from build123d import *
from build123d.topology import SkipClean

# Parameters (mm, degrees)
SKETCH3_W               = 29
SKETCH3_H               = 29
SKETCH3_R               = 1.2
SKETCH3_W_2             = 5
SKETCH3_H_2             = 6
BOSS_EXTRUDE1_DEPTH     = 5
SKETCH4_W               = 29
SKETCH4_H               = 42
SKETCH4_W_2             = 20
SKETCH4_H_2             = 11
BOSS_EXTRUDE2_DEPTH     = 10
BOSS_EXTRUDE3_START     = 3
SKETCH5_W               = 6
SKETCH5_H               = 6
SKETCH5_R               = 1.2
BOSS_EXTRUDE3_DEPTH     = 3
FILLET1_DEPTH           = 22
FILLET1_START           = 19.5
FILLET1_2_DEPTH         = 9.5
FILLET1_3_DEPTH         = 9.5
FILLET1_START_2         = 27
FILLET1_4_DEPTH         = 2
FILLET1_START_3         = 12.5
FILLET1_5_DEPTH         = 4
FILLET1_START_4         = 5
FILLET1_6_OUTLINE_R     = 1.2
FILLET1_6_DEPTH         = 20
CUT_EXTRUDE1_DEPTH      = 47.540305175
CUT_EXTRUDE1_DEPTH_BACK = 2
FILLET2_R               = 1
SKETCH7_R               = 2.05
CUT_EXTRUDE2_DEPTH      = 49.031239886
FILLET3_R               = 2


with BuildPart() as part:
    # Sketch3 → Boss-Extrude1 (new body)
    with BuildSketch(Plane.XY):
        with Locations((14.5, 14.5)):
            Rectangle(SKETCH3_W, SKETCH3_H)
        with Locations((3, 26)):
            Circle(SKETCH3_R, mode=Mode.SUBTRACT)
        with Locations(Location((26, 26, 0), (0, 0, 180))):
            Circle(SKETCH3_R, mode=Mode.SUBTRACT)
        with Locations((26, 3)):
            Circle(SKETCH3_R, mode=Mode.SUBTRACT)
        with Locations(Location((3, 3, 0), (0, 0, 180))):
            Circle(SKETCH3_R, mode=Mode.SUBTRACT)
        with Locations((24.5, 9)):
            Rectangle(SKETCH3_W_2, SKETCH3_H_2, mode=Mode.SUBTRACT)
        with BuildLine():
            Line((16.5, 7), (16.5, 22))
            ThreePointArc((16.5, 22), (18, 23.5), (19.5, 22))
            Line((19.5, 22), (19.5, 7))
            ThreePointArc((19.5, 7), (18, 5.5), (16.5, 7))
        make_face(mode=Mode.SUBTRACT)
        with BuildLine():
            Line((12.5, 7), (12.5, 22))
            ThreePointArc((12.5, 22), (11, 23.5), (9.5, 22))
            Line((9.5, 22), (9.5, 7))
            ThreePointArc((9.5, 7), (11, 5.5), (12.5, 7))
        make_face(mode=Mode.SUBTRACT)
    extrude(amount=BOSS_EXTRUDE1_DEPTH)

    # Sketch4 → Boss-Extrude2 (add)
    with BuildSketch(Plane(origin=(0, 0, 0), x_dir=(1, 0, 0), z_dir=(0, 1, 0))):
        with Locations((14.5, -4)):
            Rectangle(SKETCH4_W, SKETCH4_H)
        with Locations((14.5, 2.5)):
            Rectangle(SKETCH4_W_2, SKETCH4_H_2, mode=Mode.SUBTRACT)
    extrude(amount=-BOSS_EXTRUDE2_DEPTH)

    # Sketch5 → Boss-Extrude3 (add)
    # profile 1 of 4: a face of its own
    with BuildSketch(Plane(origin=(0, 0, 0), x_dir=(-1, 0, 0), z_dir=(0, 0, -1)).offset(BOSS_EXTRUDE3_START)):
        with Locations((-26, 3)):
            Rectangle(SKETCH5_W, SKETCH5_H)
        with Locations((-26, 3)):
            Circle(SKETCH5_R, mode=Mode.SUBTRACT)
    # profile 2 of 4: a face of its own
    with BuildSketch(Plane(origin=(0, 0, 0), x_dir=(-1, 0, 0), z_dir=(0, 0, -1)).offset(BOSS_EXTRUDE3_START)):
        with Locations((-26, 26)):
            Rectangle(SKETCH5_W, SKETCH5_H)
        with Locations((-26, 26)):
            Circle(SKETCH5_R, mode=Mode.SUBTRACT)
    # profile 3 of 4: a face of its own
    with BuildSketch(Plane(origin=(0, 0, 0), x_dir=(-1, 0, 0), z_dir=(0, 0, -1)).offset(BOSS_EXTRUDE3_START)):
        with Locations((-3, 3)):
            Rectangle(SKETCH5_W, SKETCH5_H)
        with Locations((-3, 3)):
            Circle(SKETCH5_R, mode=Mode.SUBTRACT)
    # profile 4 of 4: a face of its own
    with BuildSketch(Plane(origin=(0, 0, 0), x_dir=(-1, 0, 0), z_dir=(0, 0, -1)).offset(BOSS_EXTRUDE3_START)):
        with Locations((-3, 26)):
            Rectangle(SKETCH5_W, SKETCH5_H)
        with Locations((-3, 26)):
            Circle(SKETCH5_R, mode=Mode.SUBTRACT)
    extrude(amount=-BOSS_EXTRUDE3_DEPTH)

    # Fillet1: read off the stored shape, not the designer's step
    # Fillet1 outline → Fillet1 (add)
    with BuildSketch(Plane.YZ):
        with BuildLine():
            Line((12, 5), (12, 6.66969722))
            ThreePointArc((12, 6.66969722), (3.266799469, 14.04554885), (0, 25))
            Line((0, 25), (0, 5))
            Line((0, 5), (12, 5))
        make_face()
    extrude(amount=FILLET1_DEPTH)

    # Fillet1 2 outline → Fillet1 2 (add)
    with SkipClean():  # the faces are left unmerged after this step: merging them gives an invalid solid
        with BuildSketch(Plane.YZ.offset(FILLET1_START)):
            with BuildLine():
                ThreePointArc((20, 5), (15.913807126, 5.421873741), (12, 6.66969722))
                Line((12, 6.66969722), (12, 5))
                Line((12, 5), (20, 5))
            make_face()
            with BuildLine():
                Line((6, 5), (6, 10.717143143))
                ThreePointArc((6, 10.717143143), (1.560911085, 17.254033307), (0, 25))
                Line((0, 25), (0, 5))
                Line((0, 5), (6, 5))
            make_face()
        extrude(amount=FILLET1_2_DEPTH)
    add(part.part.scale(1), mode=Mode.REPLACE)  # the faces are merged on a copy

    # Fillet1 3 outline → Fillet1 3 (add)
    with BuildSketch(Plane.YZ):
        with BuildLine():
            ThreePointArc((20, 5), (15.913807126, 5.421873741), (12, 6.66969722))
            Line((12, 6.66969722), (12, 5))
            Line((12, 5), (20, 5))
        make_face()
    extrude(amount=FILLET1_3_DEPTH)

    # Fillet1 4 outline → Fillet1 4 (add)
    with BuildSketch(Plane.YZ.offset(FILLET1_START_2)):
        with BuildLine():
            Line((12, 5), (12, 6.66969722))
            ThreePointArc((12, 6.66969722), (8.815392066, 8.419754363), (6, 10.717143143))
            Line((6, 10.717143143), (6, 5))
            Line((6, 5), (12, 5))
        make_face()
    extrude(amount=FILLET1_4_DEPTH)

    # Fillet1 5 outline → Fillet1 5 (add)
    with SkipClean():  # the faces are left unmerged after this step: merging them gives an invalid solid
        with BuildSketch(Plane.YZ.offset(FILLET1_START_3)):
            with BuildLine():
                ThreePointArc((20, 5), (15.913807126, 5.421873741), (12, 6.66969722))
                Line((12, 6.66969722), (12, 5))
                Line((12, 5), (20, 5))
            make_face()
        extrude(amount=FILLET1_5_DEPTH)

    # Fillet1 6 outline → Fillet1 6 (cut)
    with BuildSketch(Plane.XY.offset(FILLET1_START_4)):
        with Locations((26, 3)):
            Circle(FILLET1_6_OUTLINE_R)
        with Locations((3, 3)):
            Circle(FILLET1_6_OUTLINE_R)
        with BuildLine():
            ThreePointArc((16.5, 7), (18, 5.5), (19.5, 7))
            Line((19.5, 7), (19.5, 12))
            Line((19.5, 12), (16.5, 12))
            Line((16.5, 12), (16.5, 7))
        make_face()
        with BuildLine():
            ThreePointArc((9.5, 7), (11, 5.5), (12.5, 7))
            Line((12.5, 7), (12.5, 12))
            Line((12.5, 12), (9.5, 12))
            Line((9.5, 12), (9.5, 7))
        make_face()
    extrude(amount=FILLET1_6_DEPTH, mode=Mode.SUBTRACT)

    # Sketch6 → Cut-Extrude1 (cut, two sides: drawn at the far end of the back side and taken through both)
    with BuildSketch(Plane.XY.offset(5).offset(-CUT_EXTRUDE1_DEPTH_BACK)):
        Polygon((4.385640646, 0.6), (5.771281292, 3), (4.385640646, 5.4), (1.614359354, 5.4), (0.228718708, 3), (1.614359354, 0.6), align=None)
        Polygon((24.614359354, 0.6), (27.385640646, 0.6), (28.771281292, 3), (27.385640646, 5.4), (24.614359354, 5.4), (23.228718708, 3), align=None)
        Polygon((4.385640646, 23.6), (5.771281292, 26), (4.385640646, 28.4), (1.614359354, 28.4), (0.228718708, 26), (1.614359354, 23.6), align=None)
        Polygon((27.385640646, 23.6), (28.771281292, 26), (27.385640646, 28.4), (24.614359354, 28.4), (23.228718708, 26), (24.614359354, 23.6), align=None)
    extrude(amount=CUT_EXTRUDE1_DEPTH + CUT_EXTRUDE1_DEPTH_BACK, mode=Mode.SUBTRACT)

    # Fillet2
    fillet2_edges = [part.edges().sort_by_distance(p)[0] for p in [
        (28, 6, 0),
        (26, 23, 0),
        (3, 23, 0),
        (3, 6, 0),
        (6, 3, 0),
        (6, 26, 0),
        (23, 26, 0),
        (23, 3, 0),
    ]]
    fillet(fillet2_edges, radius=FILLET2_R)

    # Sketch7 → Cut-Extrude2 (cut, through all)
    with BuildSketch(Plane.ZY):
        with Locations((-13, -5)):
            Circle(SKETCH7_R)
        with Locations((17, -5)):
            Circle(SKETCH7_R)
    extrude(amount=-CUT_EXTRUDE2_DEPTH, mode=Mode.SUBTRACT)

    # Fillet3
    # the kernel refuses this fillet: 2 mm, written as the material it takes off along each edge
    with BuildSketch(Plane(origin=(-5, -10, -17), x_dir=(0, 0, 1), z_dir=(1, 0, 0)), Plane(origin=(34, -10, 25), x_dir=(0, 0, -1), z_dir=(-1, 0, 0))) as fillet3_piece_1:
        with BuildLine():
            CenterArc((FILLET3_R, -FILLET3_R), FILLET3_R, 90, 90)
            Line((0, -FILLET3_R), (0, 0))
            Line((0, 0), (FILLET3_R, 0))
        make_face()
    extrude(amount=39, mode=Mode.SUBTRACT)
    with BuildSketch(Plane(origin=(-5, 0, -17), x_dir=(0, 0, 1), z_dir=(1, 0, 0)), Plane(origin=(34, 29, 5), x_dir=(0, 0, -1), z_dir=(-1, 0, 0))) as fillet3_piece_2:
        with BuildLine():
            CenterArc((FILLET3_R, FILLET3_R), FILLET3_R, 180, 90)
            Line((0, FILLET3_R), (0, 0))
            Line((0, 0), (FILLET3_R, 0))
        make_face()
    extrude(amount=39, mode=Mode.SUBTRACT)
    with BuildSketch(Plane(origin=(19.5, 0, 25), x_dir=(0, -1, 0), z_dir=(-1, 0, 0))) as fillet3_piece_3:
        with BuildLine():
            CenterArc((1.9089023, -2), FILLET3_R, 90, 84.784091431)
            ThreePointArc((-0.082816091, -1.818181818), (-0.02071475, -0.910033465), (0, 0))
            Line((0, 0), (1.9089023, 0))
        make_face()
    extrude(amount=24.272255751, mode=Mode.SUBTRACT)
    with BuildSketch(Plane(origin=(22, 0, 25), x_dir=(0, -1, 0), z_dir=(-1, 0, 0))) as fillet3_piece_4:
        with BuildLine():
            CenterArc((1.9089023, -2), FILLET3_R, 90, 84.784091431)
            ThreePointArc((-0.082816091, -1.818181818), (-0.02071475, -0.910033465), (0, 0))
            Line((0, 0), (1.9089023, 0))
        make_face()
    extrude(amount=2.5, mode=Mode.SUBTRACT)
    with BuildSketch(Plane(origin=(33.772255751, 0, 25), x_dir=(0, -1, 0), z_dir=(-1, 0, 0))) as fillet3_piece_5:
        with BuildLine():
            CenterArc((1.9089023, -2), FILLET3_R, 90, 84.784091436)
            ThreePointArc((-0.08281609, -1.818181818), (-0.02071475, -0.910033465), (0, 0))
            Line((0, 0), (1.9089023, 0))
        make_face()
    extrude(amount=11.772255751, mode=Mode.SUBTRACT)


solid = part.part
The listing builds one solid part. Answer for the finished solid, in the listing's coordinates (mm). A direction names the side the tool comes from. Round coordinates to 2 decimals unless told otherwise and drop trailing zeros. Order: outer loops, then holes, each group sorted by start corner. A loop starts at its lowest first (then second) coordinate and runs counter-clockwise, first axis right, second up. Notation, with made-up numbers: (-30.5, 47) -> (-23.5, 47) arc R31 ccw to (-23.5, 81) -> close; hole circle Ø6 at (72, -13.5). An arc over 180 degrees is marked (long way). Write each question's results on one line, items separated by ' | '. Start each with the question number.
Q1. Each of these flat-tipped pins is pushed along its axis until it touches: pin 1 (4 mm diameter, centred on x = 26, y = 26, fed in from +Z); pin 2 (3 mm diameter, centred on y = -2.5, z = -2, fed in from -X); pin 3 (1.8 mm diameter, centred on x = 12.5, z = 0.5, fed in from -Y); pin 4 (2 mm diameter, centred on x = 7.5, y = 24.5, fed in from -Z). Where does it stop, or does it pass through?
Q2. Find section A-A (x = 21.25). Determine the outline of the cut face in (y, z).
Q3. Straight lines are drawn through the part: probe 1 along X at (y, z) = (26, 1.95); probe 2 along X at (y, z) = (9, 5); probe 3 along X at (y, z) = (21.5, 1.5). For each, find the intervals that lie inside material, in ascending order. Write a range as from..to.
Q4. Find section D-D (x = 11.25). Determine the outline of the cut face in (y, z).
Q5. Find section C-C (y = -6.5). Determine the outline of the cut face in (x, z), then the cut area to 3 significant figures.
Q6. The mould has two halves that part along Z. Classify faces 1 (the cylindrical face through (18, 23.5, 2.5)), 2 (the flat face through (14, -5, 3)), 3 (the cylindrical face through (6.285, 3.549, -0.301)): pulls with the +Z half, pulls with the -Z half, needs draft (parallel to the pull), parting line crosses it, or undercut.
Q7. Which of the six approach directions +Z, -Z, +X, -X, +Y, -Y give full straight-line access (tool end or side, diameter ignored) to faces 4 (the cylindrical face through (27.986, 6.285, -0.301)), 5 (the flat face through (4.5, -5, -2)), 6 (the flat face through (22, 9, 4)), 7 (the flat face through (5.069, 24.783, 3.986)), 8 (the flat face through (14, -5, -8))?
Q8. Find section B-B (z = -13). Determine the outline of the cut face in (x, y).
Worked answers:
1) pin 1: stops at z = 3 | pin 2: stops at x = 0 | pin 3: stops at y = 0 | pin 4: stops at z = -0.13
2) outline: (-10, -15) arc R2 ccw to (-8, -17) -> (-2, -17) arc R2 ccw to (0, -15) -> (0, -8) -> (-10, -8) -> close; (-10, 3) -> (0, 3) -> (0, 0) -> (29, 0) -> (29, 3) arc R2 ccw to (27, 5) -> (20, 5) arc R20 cw to (0.08, 23.18) arc R2 ccw to (-1.91, 25) -> (-8, 25) arc R2 ccw to (-10, 23) -> close; hole circle Ø4.1 at (-5, -13); hole circle Ø4.1 at (-5, 17)
3) probe 1: x = 0..1.8, 4.2..24.8, 27.2..29 | probe 2: x = 0..9.5, 12.5..16.5, 19.5..22, 27..29 | probe 3: x = 0..9.5, 12.5..16.5, 19.5..29
4) outline: (-10, -15) arc R2 ccw to (-8, -17) -> (-2, -17) arc R2 ccw to (0, -15) -> (0, -8) -> (-10, -8) -> close; (-10, 3) -> (0, 3) -> (0, 0) -> (5.52, 0) -> (5.52, 11.2) arc R20 cw to (0.08, 23.18) arc R2 ccw to (-1.91, 25) -> (-8, 25) arc R2 ccw to (-10, 23) -> close; (23.48, 0) -> (29, 0) -> (29, 3) arc R2 ccw to (27, 5) -> (23.48, 5) -> close; hole circle Ø4.1 at (-5, -13); hole circle Ø4.1 at (-5, 17)
5) outline: (0, -17) -> (29, -17) -> (29, -14.4) -> (0, -14.4) -> close; (0, -11.6) -> (29, -11.6) -> (29, 15.6) -> (0, 15.6) -> close; (0, 18.4) -> (29, 18.4) -> (29, 25) -> (0, 25) -> close; hole (4.5, -8) -> (24.5, -8) -> (24.5, 3) -> (4.5, 3) -> close | area: 836 mm2
6) face 1: needs draft | face 2: undercut | face 3: pulls with the -Z half
7) face 4: -Z, +X, -X | face 5: -Y | face 6: +Z, -Z | face 7: +Z | face 8: +Y, -Y
8) outline: (0, -10) -> (29, -10) -> (29, -7.05) -> (0, -7.05) -> close; (0, -2.95) -> (29, -2.95) -> (29, 0) -> (0, 0) -> close
